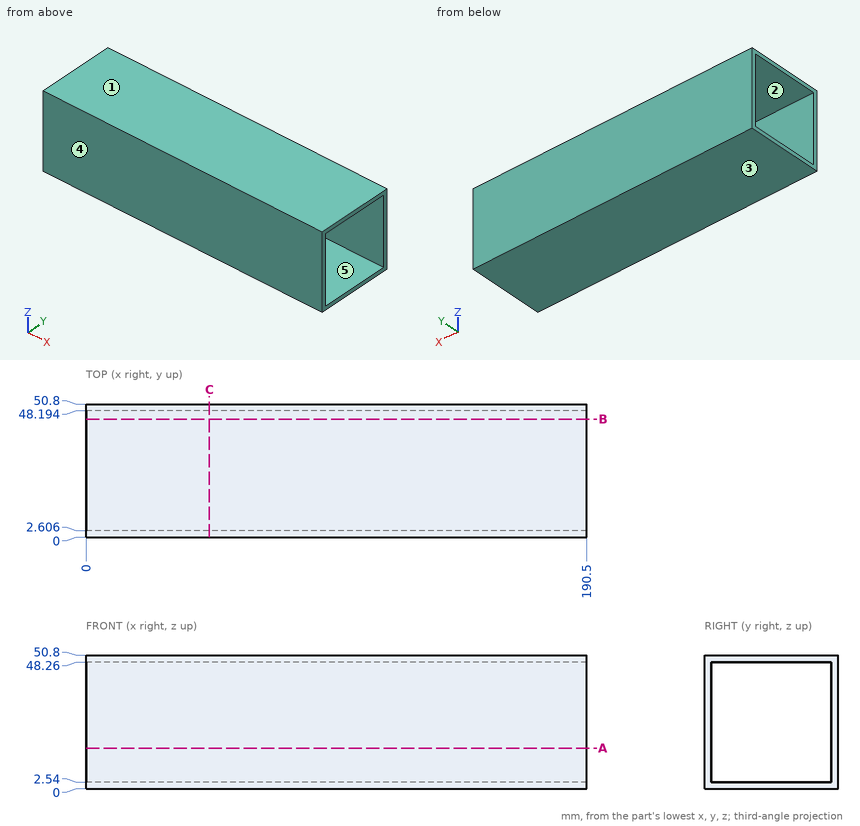
Study the drawing (mm; zero at the part's minimum x, y, z) and answer. A direction names the side the tool comes from. Give positions to 0.01 mm unless a question says otherwise; leave off trailing zeros. Write each loop counter-clockwise with the first axis right and the second up, starting at its lowest first coordinate (ties: lowest second). Pieces come first, ordered by that corner, then holes.
Item 1: Section C-C, the plane x = 47 is taken. Write down the section's boundary in (y, z).
Item 2: Section B-B, the plane y = 45 is taken. Write down the section's boundary in (x, z).
Item 3: Find the intervals of material crossed by line 1 along Y through (x, z) = (106, 9); line 2 along Z through (x, y) = (179, 31.5), in increasing order.
Item 4: Determine the mould class of the marked faces 1, 2 and 3 for opening direction Z: released by +Z, released by -Z, zero draft, split by the parting line, or undercut.
Item 5: Which of the six approach directions +Z, -Z, +X, -X, +Y, -Y give full straight-line access (tool end or side, diameter ignored) to the marked faces 4 and 5?
Item 6: Section A-A, the plane z = 15.5 is taken. Write down the section's boundary in (x, y).
Completed:
1. outline: (0, 0) - (50.8, 0) - (50.8, 50.8) - (0, 50.8) - close; hole (2.61, 2.54) - (48.19, 2.54) - (48.19, 48.26) - (2.61, 48.26) - close
2. outline: (0, 0) - (190.5, 0) - (190.5, 2.54) - (0, 2.54) - close; (0, 48.26) - (190.5, 48.26) - (190.5, 50.8) - (0, 50.8) - close
3. line 1: y = 0 to 2.61, 48.19 to 50.8
3. line 2: z = 0 to 2.54, 48.26 to 50.8
4. face 1: released by +Z
4. face 2: undercut
4. face 3: released by -Z
5. face 4: +Z, -Z, +X, -X, -Y
5. face 5: +X, -X
6. outline: (0, 0) - (190.5, 0) - (190.5, 2.61) - (0, 2.61) - close; (0, 48.19) - (190.5, 48.19) - (190.5, 50.8) - (0, 50.8) - close
